Source: three-view drawing plus pictorial views. Frame: mm from the lowest corner of the part. Give positions to 0.01 mm unless a question says otherwise; leave off trailing zeros. Loops run counter-clockwise (first coordinate to the right, second up) from the corner with the lowest first, then second, coordinate; pieces in that order, holes last. Notation, with made-up numbers: M -36,66 L -23,66 A23 ccw -23,75 Z; hole C 45,13.25 d7. An arc over 180 degrees is marked long. Answer as a JSON object with one key per item and string values. Group by question number.
1) First-contact query: P1, Ø2.5, axis at x = 47.195, z = 97.54, coming from the +Y side; P2, Ø1.5, axis at y = 1.5, z = 57.5, coming from the -X side. Flat tips, straight axial feed; report the tip coordinate or a pass-through.
2) Section query A-A on x = 5.5. Return loops of the section in (y, z).
3) Ray query, L1, parallel to X at y = 1.75, z = 5.5; L2, parallel to Z at x = 54.5, y = 0.6; L3, parallel to X at y = 0.9, z = 98. Return the intervals inside material, ascending.
4) Section query B-B on z = 5.5. Return loops of the section in (x, y), plus the area to 3 significant figures.
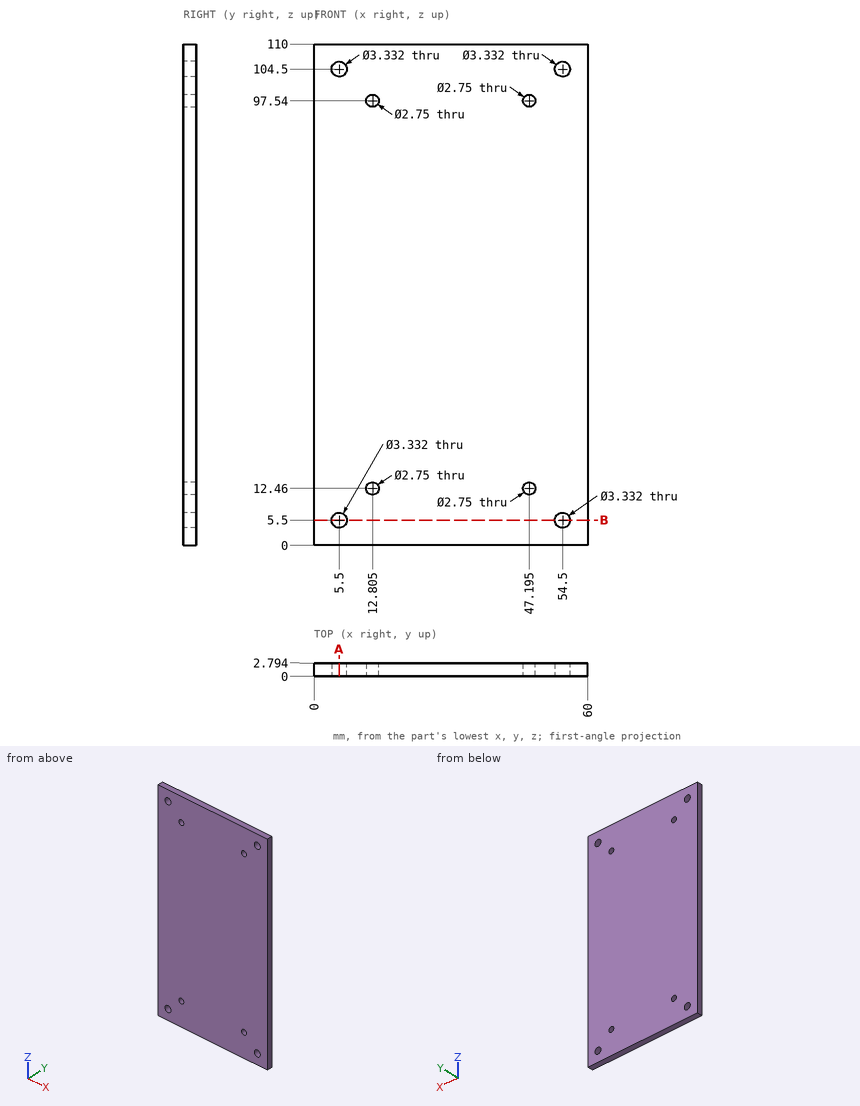
Output:
{
 "1": {"P1": "passes through", "P2": "stops at x = 0"},
 "2": {"outline": "M 0,0 L 2.79,0 L 2.79,3.83 L 0,3.83 Z; M 0,7.17 L 2.79,7.17 L 2.79,102.83 L 0,102.83 Z; M 0,106.17 L 2.79,106.17 L 2.79,110 L 0,110 Z"},
 "3": {"L1": "x = 0 to 3.83, 7.17 to 52.83, 56.17 to 60", "L2": "z = 0 to 3.83, 7.17 to 102.83, 106.17 to 110", "L3": "x = 0 to 11.51, 14.1 to 45.9, 48.49 to 60"},
 "4": {"outline": "M 0,0 L 3.83,0 L 3.83,2.79 L 0,2.79 Z; M 7.17,0 L 52.83,0 L 52.83,2.79 L 7.17,2.79 Z; M 56.17,0 L 60,0 L 60,2.79 L 56.17,2.79 Z", "area": "149 mm^2"}
}
